Work out the finished part from the listing and answer in its coordinate system (mm). Face numbers are marked on the shaded views. A direction names the side the tool comes from. Give positions to 0.01 mm unless a question says otherwise; leave off trailing zeros. Loops run counter-clockwise (first coordinate to the right, second up) from the corner with the lowest first, then second, coordinate; pieces in that order, holes last. Notation, with made-up numbers: M 51,45.25 L 85,45.25 A17 cw 85,71.25 Z; hole C 77.5,82 d7. An arc over 180 degrees is marked long. Write item = value, one per line. Start each with the question number.
1. Section D-D on y = 6.5 is taken. Determine the outline of the cut face in (x, z).
2. For the marked faces 5 and 6, determine the directions among +Z, -Z, +X, -X, +Y, -Y from which every point of the face is accessible in a straight line to the end or side of a thin tool.
3. Section B-B on x = 0 is taken. Determine the outline of the cut face in (y, z), plus the area to 3 significant figures.
4. Flat-ended cylindrical pins translate along their axes: pin 1 Ø1.5 at (x, y) = (5, 1.5) entering from -Z; pin 2 Ø3 at (y, z) = (11, -6) entering from -X; pin 3 Ø2 at (y, z) = (6.5, 0) entering from +X. Find the tip coordinate at first contact, or state that the pin passes through.
5. Consider L1, parallel to Z at x = 4.75, y = 6.5; L2, parallel to X at y = 4.25, z = 0; L3, parallel to Z at x = -3.75, y = 11.25. Determine where each line is inside the solid, lowest interval first. Write a range as [from, to].
6. Section C-C on x = -3.5 is taken. Determine the outline of the cut face in (y, z), plus the area to 3 significant figures.
7. The mould has two halves that part along Z. Classify the marked faces 1, 2, 3 and 4: released by +Z, released by -Z, zero draft, split by the parting line, or undercut.
8. Section A-A on z = 0 is taken. Determine the outline of the cut face in (x, y), plus the area to 3 significant figures.
```python
from build123d import *

# Parameters (mm, degrees)
SKETCH_1_R          = 8
SKETCH_1_R_2        = 1.25
EXTRUDE_1_DEPTH     = 12.5
SKETCH_3_R          = 1.75
CUT_EXTRUDE_1_DEPTH = 10


with BuildPart() as part:
    # 草图1 → 凸台-拉伸1 (new body)
    with BuildSketch(Plane(origin=(0, 0, 0), x_dir=(1, 0, 0), z_dir=(0, 1, 0))):
        with Locations(Location((0, 0, 0), (0, 0, 270))):
            Circle(SKETCH_1_R)
        with Locations(Location((4.242640687, 4.242640687, 0), (0, 0, 270))):
            Circle(SKETCH_1_R_2, mode=Mode.SUBTRACT)
        with Locations(Location((4.242640687, -4.242640687, 0), (0, 0, 270))):
            Circle(SKETCH_1_R_2, mode=Mode.SUBTRACT)
        with Locations(Location((-4.242640687, -4.242640687, 0), (0, 0, 270))):
            Circle(SKETCH_1_R_2, mode=Mode.SUBTRACT)
        with Locations(Location((-4.242640687, 4.242640687, 0), (0, 0, 270))):
            Circle(SKETCH_1_R_2, mode=Mode.SUBTRACT)
        with BuildLine():
            Line((2.5, 1.658312395), (2.5, -1.658312395))
            ThreePointArc((2.5, -1.658312395), (-3, 0), (2.5, 1.658312395))
        make_face(mode=Mode.SUBTRACT)
    extrude(amount=EXTRUDE_1_DEPTH)

    # 草图3 → 切除-拉伸1 (cut)
    with BuildSketch(Plane.ZY.offset(-2.5)):
        with Locations((0, 6.5)):
            Circle(SKETCH_3_R)
    extrude(amount=-CUT_EXTRUDE_1_DEPTH, mode=Mode.SUBTRACT)


solid = part.part
```
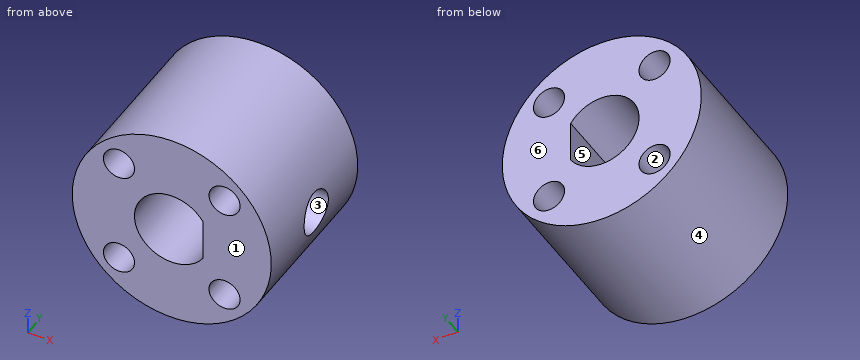
Verdict:
q1.outline = M 2.5,-1.75 L 2.5,-1.66 A3 cw long 2.5,1.66 L 2.5,1.75 L 7.81,1.75 A8 ccw long 7.81,-1.75 Z; hole C -4.24,-4.24 d2.5; hole C -4.24,4.24 d2.5; hole C 4.24,-4.24 d2.5; hole C 4.24,4.24 d2.5
q2.face_5 = +Y, -Y
q2.face_6 = +Z, -Z, +X, -X, +Y
q3.outline = M 0,-8 L 12.5,-8 L 12.5,-3 L 0,-3 Z; M 0,3 L 12.5,3 L 12.5,8 L 0,8 Z
q3.area = 125 mm2
q4.pin_1 = -6.78
q4.pin_2 = -6.61
q4.pin_3 = -2.83
q5.L1 = [-6.44, -5.39], [-3.1, -1.75], [1.75, 3.1], [5.39, 6.44]
q5.L2 = [-8, -3], [2.5, 8]
q5.L3 = [-7.07, -5.39], [-3.09, 3.09], [5.39, 7.07]
q6.outline = M 0,-7.19 L 12.5,-7.19 L 12.5,-5.25 L 0,-5.25 Z; M 0,-3.24 L 12.5,-3.24 L 12.5,3.24 L 0,3.24 Z; M 0,5.25 L 12.5,5.25 L 12.5,7.19 L 0,7.19 Z
q6.area = 130 mm2
q7.face_1 = zero draft
q7.face_2 = undercut
q7.face_3 = undercut
q7.face_4 = split by the parting line
q8.outline = M -8,0 L -3,0 L -3,12.5 L -8,12.5 Z; M 2.5,0 L 8,0 L 8,4.75 L 2.5,4.75 Z; M 2.5,8.25 L 8,8.25 L 8,12.5 L 2.5,12.5 Z
q8.area = 112 mm2
